```python
from build123d import *

# Parameters (mm, degrees)
F0_W     = 622.3
F0_H     = 501.65
F1_DEPTH = 25.4
F2_T     = -2.54
F3_W     = 34.925
F3_H     = 82.55
F3_R     = 2.579688
F3_R_2   = 3.175
F4_DEPTH = 50.801
F5_R     = 2.5781
F6_DEPTH = 501.651


with BuildPart() as f1:
    # F0 (on Top) → F1 (new body, symmetric)
    with BuildSketch(Plane.XY):
        Rectangle(F0_W, F0_H)
    extrude(amount=F1_DEPTH, both=True)

    # F2
    f2_openings = [f1.faces().sort_by_distance(p)[0] for p in [
        (0, 0, -25.4),
    ]]
    offset(amount=F2_T, openings=f2_openings)

    # F3 (on face) → F4 (cut, through all)
    with BuildSketch(Plane.XY.offset(25.4)):
        with Locations((-293.6875, -209.55)):
            Rectangle(F3_W, F3_H)
        with Locations((293.6875, -209.55)):
            Rectangle(F3_W, F3_H)
        with Locations((174.244, -0.762)):
            Circle(F3_R)
        with Locations((-174.244, -0.762)):
            Circle(F3_R)
        with Locations((-160.909, -244.475)):
            Circle(F3_R)
        with Locations((160.909, -244.475)):
            Circle(F3_R)
        with Locations((-298.45, 225.425)):
            Circle(F3_R_2)
        with Locations((-298.45, 41.275)):
            Circle(F3_R_2)
        with Locations((-298.45, -142.875)):
            Circle(F3_R_2)
        with Locations((298.45, -142.875)):
            Circle(F3_R_2)
        with Locations((298.45, 41.275)):
            Circle(F3_R_2)
        with Locations((298.45, 225.425)):
            Circle(F3_R_2)
    extrude(amount=-F4_DEPTH, mode=Mode.SUBTRACT)

    # F5 (on face) → F6 (cut, through all)
    with BuildSketch(Plane.XZ.offset(250.825)):
        Circle(F5_R)
        with Locations((125.4125, 0)):
            Circle(F5_R)
        with Locations((250.825, 0)):
            Circle(F5_R)
        with Locations((-125.4125, 0)):
            Circle(F5_R)
        with Locations((-250.825, 0)):
            Circle(F5_R)
    extrude(amount=-F6_DEPTH, mode=Mode.SUBTRACT)


solid = f1.part
```
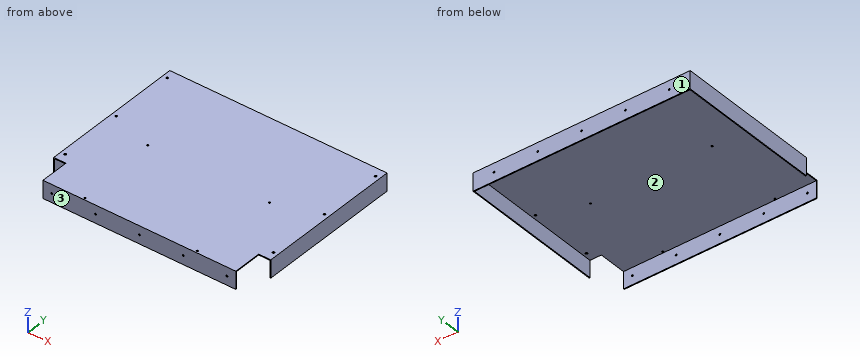
Here's how the part is built. I have some questions about the finished solid (model axes, mm). Face numbers are marked on the shaded views. Round coordinates to 2 decimals unless told otherwise and drop trailing zeros. Write each loop counter-clockwise with the first axis right and the second up, starting at its lowest first coordinate (ties: lowest second). Pieces come first, ordered by that corner, then holes.
Q1. If we section it at B-B on y = 52.5: Write out the boundary of the cut face in (x, z), plus the area to 3 significant figures.
Q2. Will these pins go through, and if not, where does the flat tip stop? P1, Ø5, axis at x = -298.45, y = 41.275, coming from the -Z side; P2, Ø6, axis at x = 140.5, y = 16.5, coming from the -Z side.
Q3. If we section it at A-A on z = 11: Write out the boundary of the cut face in (x, y) (3 decimals), plus the area to 3 significant figures.
Q4. If we section it at C-C on x = -64: Write out the boundary of the cut face in (y, z) (3 decimals), plus the area to 3 significant figures.
Q5. If we mould it in two halves opening along Y, with no side actions, what happens to the marked faces 1, 2 and 3? For each: +Y half, -Y half, draft (parallel to the pull), parting line (faces both ways), or undercut.
Q6. Please list where these lines run through material, in increasing order: probe 1 along Y at (x, z) = (298, 23) (3 decimals); probe 2 along X at (y, z) = (-166, -18); probe 3 along Y at (x, z) = (190, -9) (3 decimals).
Answer below:
1. outline: (-311.15, -25.4) - (-308.61, -25.4) - (-308.61, 22.86) - (308.61, 22.86) - (308.61, -25.4) - (311.15, -25.4) - (311.15, 25.4) - (-311.15, 25.4) - close
1. area: 1,830 mm2
2. P1: passes through
2. P2: stops at z = 22.86
3. outline: (-311.15, -168.275) - (-308.61, -168.275) - (-308.61, 248.285) - (308.61, 248.285) - (308.61, -168.275) - (311.15, -168.275) - (311.15, 250.825) - (-311.15, 250.825) - close; (-276.225, -250.825) - (276.225, -250.825) - (276.225, -248.285) - (-276.225, -248.285) - close
3. area: 5,100 mm2
4. outline: (-250.825, -25.4) - (-248.285, -25.4) - (-248.285, 22.86) - (248.285, 22.86) - (248.285, -25.4) - (250.825, -25.4) - (250.825, 25.4) - (-250.825, 25.4) - close
4. area: 1,520 mm2
5. face 1: +Y half
5. face 2: undercut
5. face 3: -Y half
6. probe 1: y = -168.275 to -146.018, -139.732 to 38.132, 44.418 to 222.282, 228.568 to 250.825
6. probe 2: x = -311.15 to -308.61, 308.61 to 311.15
6. probe 3: y = -250.825 to -248.285, 248.285 to 250.825
